For this review, take the finished solid that the model builds, in its own axes (mm). Face numbers are marked on the shaded views. A direction names the side the tool comes from. Give positions to 0.01 mm unless a question says otherwise; leave off trailing zeros. Loops run counter-clockwise (first coordinate to the right, second up) from the corner with the lowest first, then second, coordinate; pieces in that order, holes last. Notation, with made-up numbers: (25, 21.25) -> (36, 21.25) arc R25 cw to (36, 43.25) -> close; hole circle Ø7 at (49.25, -24). An arc over 180 degrees is marked (long way). One line per question, with ' | ' between items. Start each with the question number.
(1) Tool access review of the marked faces 1 and 2: name each direction out of +Z, -Z, +X, -X, +Y, -Y from which nothing blocks a thin tool from reaching the whole face with its end or side.
(2) Wall thickness on probe 1 along Z at (x, y) = (80.25, 6.25); probe 2 along Z at (x, y) = (35.5, 4.5); probe 3 along X at (y, z) = (0.5, 44): over which ranges is each line inside the solid? List them lowest first.
(3) Consider section D-D (x = 50). Write out the cut boundary in (y, z), and give its area (3 significant figures).
(4) Consider section B-B (y = 6.75). Write out the cut boundary in (x, z).
(5) Consider section A-A (x = 17.8). Write out the cut boundary in (y, z).
(6) Insertion check: P1, Ø4, axis at y = 3.5, z = 51.5, coming from the -X side; P2, Ø1.5, axis at x = 66, y = 2.5, coming from the -Z side; P3, Ø2.5, axis at x = -7.5, y = 1.5, coming from the -Z side; P4, Ø3.5, axis at x = 35.4, z = 15, coming from the -Y side. Each pin has a flat end and moves straight along its axis. Give the tip position at first contact, or say it passes through.
(7) Consider section C-C (z = 132). Write out the cut boundary in (x, y), and give its area (3 significant figures).
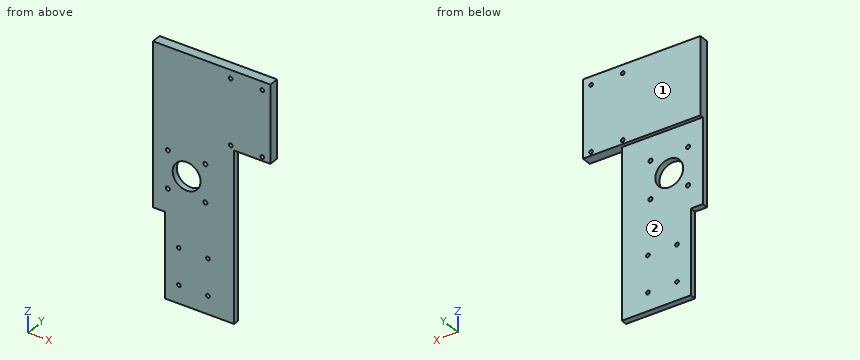
from build123d import *

# Parameters (mm, degrees)
SKETCH_1_W               = 57
SKETCH_1_H               = 140
EXTRUDE_1_DEPTH          = 5
SKETCH_2_R               = 1.55
CUT_EXTRUDE_1_DEPTH      = 10
SKETCH_5_W               = 70
SKETCH_5_H               = 5
EXTRUDE_2_DEPTH          = 10
SKETCH_6_R               = 11.5
SKETCH_6_R_2             = 1.7
CUT_EXTRUDE_2_DEPTH      = 10
EXTRUDE_4_DEPTH          = 3
EXTRUDE_4_DEPTH_BACK     = 5
CUT_EXTRUDE_3_DEPTH      = 222.921157171
CUT_EXTRUDE_3_DEPTH_BACK = 222.921157171
SKETCH_8_R               = 1.55


with BuildPart() as part:
    # 草图1 → 凸台-拉伸1 (new body)
    with BuildSketch(Plane(origin=(0, 0, 0), x_dir=(1, 0, 0), z_dir=(0, 1, 0))):
        with Locations((28.5, -70)):
            Rectangle(SKETCH_1_W, SKETCH_1_H)
    extrude(amount=EXTRUDE_1_DEPTH)

    # 草图2 → 切除-拉伸1 (cut)
    with BuildSketch(Plane.XZ):
        with Locations(Location((11.4, 45, 0), (0, 0, 270))):
            Circle(SKETCH_2_R)
        with Locations(Location((11.4, 15, 0), (0, 0, 270))):
            Circle(SKETCH_2_R)
        with Locations(Location((35.4, 15, 0), (0, 0, 270))):
            Circle(SKETCH_2_R)
        with Locations(Location((35.4, 45, 0), (0, 0, 270))):
            Circle(SKETCH_2_R)
    extrude(amount=-CUT_EXTRUDE_1_DEPTH, mode=Mode.SUBTRACT)

    # 草图5 → 凸台-拉伸2 (add)
    with BuildSketch(Plane.ZY):
        with Locations((105, 2.5)):
            Rectangle(SKETCH_5_W, SKETCH_5_H)
    extrude(amount=EXTRUDE_2_DEPTH)

    # 草图6 → 切除-拉伸2 (cut)
    with BuildSketch(Plane(origin=(0, 5, 0), x_dir=(1, 0, 0), z_dir=(0, 1, 0))):
        with Locations(Location((17.8, -105, 0), (0, 0, 270))):
            Circle(SKETCH_6_R)
        with Locations(Location((33.3, -89.5, 0), (0, 0, 270))):
            Circle(SKETCH_6_R_2)
        with Locations(Location((2.3, -89.5, 0), (0, 0, 270))):
            Circle(SKETCH_6_R_2)
        with Locations(Location((2.3, -120.5, 0), (0, 0, 270))):
            Circle(SKETCH_6_R_2)
        with Locations(Location((33.3, -120.5, 0), (0, 0, 270))):
            Circle(SKETCH_6_R_2)
    extrude(amount=-CUT_EXTRUDE_2_DEPTH, mode=Mode.SUBTRACT)

    # 草图7 → 凸台-拉伸4 (add, two sides: drawn at the far end of the back side and taken through both)
    with BuildSketch(Plane(origin=(0, 5, 0), x_dir=(1, 0, 0), z_dir=(0, 1, 0)).offset(-EXTRUDE_4_DEPTH_BACK)):
        Polygon((87, -140), (57, -140), (-10, -140), (-10, -204), (87, -204), align=None)
    extrude(amount=EXTRUDE_4_DEPTH + EXTRUDE_4_DEPTH_BACK)

    # 草图8 → 切除-拉伸3 (cut, two sides: drawn at the far end of the back side and taken through both)
    with BuildSketch(Plane.XZ.offset(-CUT_EXTRUDE_3_DEPTH_BACK)):
        with Locations(Location((54.15, 197.137921192, 0), (0, 0, 270))):
            Circle(SKETCH_8_R)
        with Locations(Location((80.25, 197.137921192, 0), (0, 0, 270))):
            Circle(SKETCH_8_R)
        with Locations(Location((54.15, 143.137921192, 0), (0, 0, 270))):
            Circle(SKETCH_8_R)
        with Locations(Location((80.25, 143.137921192, 0), (0, 0, 270))):
            Circle(SKETCH_8_R)
    extrude(amount=CUT_EXTRUDE_3_DEPTH + CUT_EXTRUDE_3_DEPTH_BACK, mode=Mode.SUBTRACT)


solid = part.part
A:
1) face 1: +Z, -Z, +X, -X, +Y | face 2: -Z, +X, -X, +Y
2) probe 1: z = 140 to 141.59, 144.69 to 195.59, 198.69 to 204 | probe 2: z = 0 to 13.45, 16.55 to 43.45, 46.55 to 204 | probe 3: x = 0 to 10.22, 12.58 to 34.22, 36.58 to 57
3) outline: (0, 0) -> (5, 0) -> (5, 140) -> (8, 140) -> (8, 204) -> (0, 204) -> close | area: 1,210 mm^2
4) outline: (-10, 140) -> (87, 140) -> (87, 204) -> (-10, 204) -> close; hole circle Ø3.1 at (54.15, 143.14); hole circle Ø3.1 at (54.15, 197.14); hole circle Ø3.1 at (80.25, 143.14); hole circle Ø3.1 at (80.25, 197.14)
5) outline: (0, 0) -> (5, 0) -> (5, 93.5) -> (0, 93.5) -> close; (0, 116.5) -> (5, 116.5) -> (5, 140) -> (8, 140) -> (8, 204) -> (0, 204) -> close
6) P1: stops at x = 0 | P2: stops at z = 140 | P3: stops at z = 70 | P4: stops at y = 0
7) outline: (-10, 0) -> (57, 0) -> (57, 5) -> (-10, 5) -> close | area: 335 mm^2
